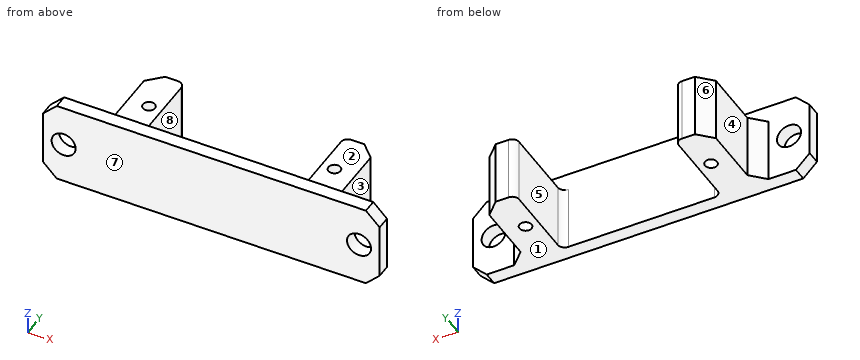
```python
from build123d import *

# Parameters (mm, degrees)
F0_W     = 8
F0_H     = 2
F1_DEPTH = 12
F0_W_2   = 4.875
F0_H_2   = 12.5
F0_R     = 0.875
F2_DEPTH = 9.5
F3_SIZE  = 2
F4_R     = 1.75
F5_DEPTH = 2
F6_R     = 1


with BuildPart() as f1:
    # F0 (on Top) → F1 (new body)
    with BuildSketch(Plane.XY):
        Polygon((-11.625, -5.25), (-16.5, -5.25), (-16.5, -7.25), (16.5, -7.25), (16.5, -5.25), (11.625, -5.25), align=None)
        with Locations((-20.5, -6.25)):
            Rectangle(F0_W, F0_H)
        with Locations((20.5, -6.25)):
            Rectangle(F0_W, F0_H)
    extrude(amount=F1_DEPTH)

    # F0 (on Top) → F2 (join)
    with BuildSketch(Plane.XY):
        with Locations((-14.0625, 1)):
            Rectangle(F0_W_2, F0_H_2)
        with Locations((-13.5, 1)):
            Circle(F0_R, mode=Mode.SUBTRACT)
        with Locations((14.0625, 1)):
            Rectangle(F0_W_2, F0_H_2)
        with Locations((13.5, 1)):
            Circle(F0_R, mode=Mode.SUBTRACT)
    extrude(amount=F2_DEPTH)

    # F3
    f3_edges = [f1.edges().sort_by_distance(p)[0] for p in [
        (-16.5, 7.25, 4.75),
        (16.5, 7.25, 4.75),
        (-24.5, -6.25, 12),
        (-24.5, -6.25, 0),
        (24.5, -6.25, 12),
        (24.5, -6.25, 0),
        (-16.5, -5.25, 4.75),
        (16.5, -5.25, 4.75),
    ]]
    chamfer(f3_edges, length=F3_SIZE)

    # F4 (on face) → F5 (cut, through all)
    with BuildSketch(Plane(origin=(0, -5.25, 0), x_dir=(-1, 0, 0), z_dir=(0, 1, 0))):
        with Locations((21.5, 6)):
            Circle(F4_R)
        with Locations((-21.5, 6)):
            Circle(F4_R)
    extrude(amount=-F5_DEPTH, mode=Mode.SUBTRACT)

    # F6
    f6_edges = [f1.edges().sort_by_distance(p)[0] for p in [
        (11.625, -5.25, 4.75),
        (-11.625, -5.25, 4.75),
        (-11.625, 7.25, 4.75),
        (11.625, 7.25, 4.75),
    ]]
    fillet(f6_edges, radius=F6_R)


solid = f1.part
```
Geometry check sheet. Reference: the model listing, model coordinates, mm. Face numbers are marked on the shaded views. A direction names the side the tool comes from. Round coordinates to 2 decimals unless told otherwise and drop trailing zeros. Write each loop counter-clockwise with the first axis right and the second up, starting at its lowest first coordinate (ties: lowest second). Pieces come first, ordered by that corner, then holes. Notation, with made-up numbers: (-1.5, -10) - (5.5, -10) arc R5 ccw to (5.5, -3) - close; hole circle Ø5 at (78.5, 5.5). An arc over 180 degrees is marked (long way). Write each question's results on one line, items separated by ' | '.
(1) Sectioned sample at A-A, the plane y = 1. Enter the section's corners in (x, z) (3 decimals).
Computed:
outline: (-16.5, 0) - (-14.375, 0) - (-14.375, 9.5) - (-16.5, 9.5) - close; (-12.625, 0) - (-11.625, 0) - (-11.625, 9.5) - (-12.625, 9.5) - close; (11.625, 0) - (12.625, 0) - (12.625, 9.5) - (11.625, 9.5) - close; (14.375, 0) - (16.5, 0) - (16.5, 9.5) - (14.375, 9.5) - close
(2) Draft check along X on the marked faces 6, 7 and 8. Enter one of: pulls with the +X half, pulls with the -X half, needs draft (parallel to the pull), parting line crosses it, or undercut.
Computed:
face 6: pulls with the -X half | face 7: needs draft | face 8: undercut
(3) Set-up check for the marked faces 1, 2, 3, 4 and 5: record each of +Z, -Z, +X, -X, +Y, -Y from which the full face is reachable in a straight line by a thin tool's end or side.
Computed:
face 1: -Z, +X, -X, +Y, -Y | face 2: +Z, +X, -X, +Y | face 3: +Z, -Z, +X, +Y | face 4: +Z, -Z, -X, +Y | face 5: +Z, -Z, +Y
(4) Sectioned sample at D-D, the plane z = 6.75. Count the separate pieces of the cut face and the enclosed holes in it, plus the area to 3 significant figures.
Computed:
separate pieces: 3 | enclosed holes: 2 | area: 202 mm^2
(5) Depth check by flat-ended pin: pin 1 Ø5 at (y, z) = (-4, 8) entering from +X; pin 2 Ø3 at (y, z) = (2.5, 3.5) entering from +X; pin 3 Ø2 at (x, y) = (15, -1) entering from +Z; pin 4 Ø6 at (y, z) = (-1, 7) entering from -X. Enter the tip coordinate at first touch or a pass-through.
Computed:
pin 1: stops at x = 24.5 | pin 2: stops at x = 16.5 | pin 3: stops at z = 9.5 | pin 4: stops at x = -17.25
(6) Sectioned sample at B-B, the plane x = 21.5. Enter the section's corners in (y, z), plus the area to 3 significant figures.
Computed:
outline: (-7.25, 0) - (-5.25, 0) - (-5.25, 4.25) - (-7.25, 4.25) - close; (-7.25, 7.75) - (-5.25, 7.75) - (-5.25, 12) - (-7.25, 12) - close | area: 17.0 mm^2
(7) Sectioned sample at C-C, the plane z = 3.5. Enter the section's corners in (x, y) (3 decimals).
Computed:
outline: (-24.5, -7.25) - (24.5, -7.25) - (24.5, -5.25) - (18.5, -5.25) - (16.5, -3.25) - (16.5, 5.25) - (14.5, 7.25) - (12.625, 7.25) arc R1 ccw to (11.625, 6.25) - (11.625, -4.25) arc R1 cw to (10.625, -5.25) - (-10.625, -5.25) arc R1 cw to (-11.625, -4.25) - (-11.625, 6.25) arc R1 ccw to (-12.625, 7.25) - (-14.5, 7.25) - (-16.5, 5.25) - (-16.5, -3.25) - (-18.5, -5.25) - (-24.5, -5.25) - close; hole circle Ø1.75 at (-13.5, 1); hole circle Ø1.75 at (13.5, 1)
(8) Thickness scan on probe 1 along Y at (x, z) = (-13.5, 3) (3 decimals); probe 2 along X at (y, z) = (-2, 7) (3 decimals); probe 3 along Z at (x, y) = (21.5, -5.7). Record the ranges inside material, lowest first. Write a range as from..to.
Computed:
probe 1: y = -7.25..0.125, 1.875..7.25 | probe 2: x = -16.5..-11.625, 11.625..16.5 | probe 3: z = 0..4.25, 7.75..12
